Part model, mm, in its own coordinate system. Round coordinates to 2 decimals unless told otherwise and drop trailing zeros. Write each loop counter-clockwise with the first axis right and the second up, starting at its lowest first coordinate (ties: lowest second). Pieces come first, ordered by that corner, then holes. Notation, with made-up numbers: M -25,1 L -19,1 A13 cw -19,15 Z; hole C -32.75,4.25 d11. An arc over 180 degrees is marked long. One line per question, with ' | ' between items. Start each with the question number.
1) Saw through at B-B (y = 4.75). List the corners of the cut face in (x, z), plus the area to 3 significant figures.
2) Drop flat-ended pins along their axis: pin 1 Ø5 at (x, z) = (-0.5, -46) entering from +Y; pin 2 Ø1.8 at (y, z) = (7, -14) entering from +X; pin 3 Ø3 at (x, y) = (0, 3.5) entering from -Z. Give the stop position or say it passes through.
3) Wall check: probe 1 along X at (y, z) = (0.5, -31); probe 2 along Y at (x, z) = (-4.5, -27.5); probe 3 along Y at (x, z) = (0.5, -66.5). Give the ranges that are in metal, low to high. Write a range as [from, to].
4) Saw through at A-A (z = -34). List the corners of the cut face in (x, y), plus the area to 3 significant figures.
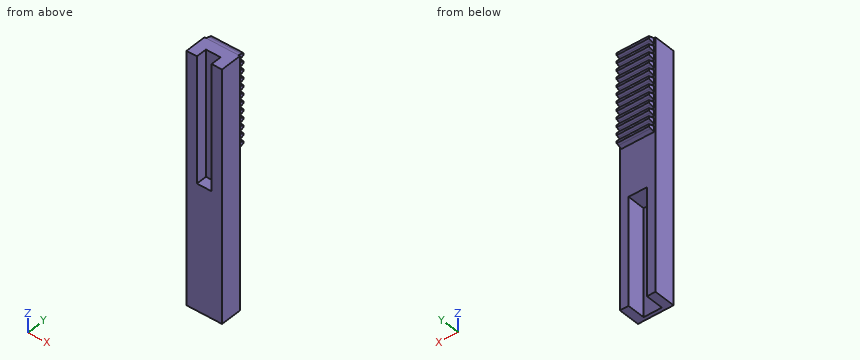
```python
from build123d import *

# Parameters (mm, degrees)
SKETCH_2_W             = 70
SKETCH_2_H             = 6
EXTRUDE_2_DEPTH        = 4.95
EXTRUDE_3_DEPTH        = 4.5
PATTERN_LINEAR_1_COUNT = 12
PATTERN_LINEAR_1_PITCH = 2.2
SKETCH_7_W             = 5.1
SKETCH_7_H             = 30
CUT_EXTRUDE_1_DEPTH    = 5
SKETCH_3_W             = 35
SKETCH_3_H             = 3
CUT_EXTRUDE_2_DEPTH    = 2.05


with BuildPart() as part:
    # Sketch 2 → Extrude 2 (new, symmetric)
    with BuildSketch(Plane(origin=(0, 0, 0), x_dir=(0, 0, -1), z_dir=(1, 0, 0))):
        with Locations((35, 3)):
            Rectangle(SKETCH_2_W, SKETCH_2_H)
    extrude(amount=EXTRUDE_2_DEPTH, both=True)

    # Sketch 2_4 → Extrude 3 (add, symmetric)
    with BuildSketch(Plane(origin=(0, 0, 0), x_dir=(0, 0, -1), z_dir=(1, 0, 0))):
        Polygon((0.291798614, 7.03781361), (0, 6), (1.6, 6), (1.308201386, 7.03781361), align=None)
        Polygon((0.291798614, 7.03781361), (0.475, 7.7), (1.125, 7.7), (1.308201386, 7.03781361), align=None)
    extrude_3 = extrude(amount=EXTRUDE_3_DEPTH, both=True)

    # Pattern Linear 1: Extrude 3 ×12
    with Locations(*[(0, 0, -i * PATTERN_LINEAR_1_PITCH) for i in range(1, PATTERN_LINEAR_1_COUNT)]):
        add(extrude_3)

    # Sketch 7 → Cut-Extrude 1 (cut)
    with BuildSketch(Plane(origin=(0, 6, 0), x_dir=(1, 0, 0), z_dir=(0, 1, 0))):
        with Locations((0, 55)):
            Rectangle(SKETCH_7_W, SKETCH_7_H)
    extrude(amount=-CUT_EXTRUDE_1_DEPTH, mode=Mode.SUBTRACT)

    # Sketch 3 → Cut-Extrude 2 (cut, symmetric)
    with BuildSketch(Plane(origin=(0, 0, 0), x_dir=(0, 0, -1), z_dir=(1, 0, 0))):
        with Locations((17.5, 1.5)):
            Rectangle(SKETCH_3_W, SKETCH_3_H)
    extrude(amount=CUT_EXTRUDE_2_DEPTH, both=True, mode=Mode.SUBTRACT)


solid = part.part
```
Answer key:
1) outline: M -4.95,-70 L -2.55,-70 L -2.55,-40 L 2.55,-40 L 2.55,-70 L 4.95,-70 L 4.95,0 L -4.95,0 Z | area: 540 mm2
2) pin 1: stops at y = 6 | pin 2: stops at x = 4.5 | pin 3: stops at z = -40
3) probe 1: x = [-4.95, -2.05], [2.05, 4.95] | probe 2: y = [0, 6] | probe 3: y = [0, 1]
4) outline: M -4.95,0 L -2.05,0 L -2.05,3 L 2.05,3 L 2.05,0 L 4.95,0 L 4.95,6 L -4.95,6 Z | area: 47.1 mm2
